Part model, mm, in its own coordinate system. A direction names the side the tool comes from. Coordinates: 2 decimals unless noted, no trailing zeros. Loops run counter-clockwise (first coordinate to the right, second up) from the corner with the lowest first, then second, coordinate; pieces in that order, holes last. Notation, with made-up numbers: (-16, 21.5) - (40, 21.5) arc R23 ccw to (40, 31.5) - close; hole circle Ø11 at (42, 85.5). An arc over 180 degrees is marked (long way). Use a Markdown table: item, result. Add a question column.
1) Tool access for faces 4 (the face through (0, 0, -2)), 5 (the face through (5, 0, -1.27)), 6 (the face through (4, 0, 0)): list every direction of +Z, -Z, +X, -X, +Y, -Y with a clear straight run to the whole face (end or side of a thin tool).
2) Band-saw the part on A-A (z = -2). Give the cut face in (x, y).
3) Drop flat-ended pins along their axis: P1, Ø8, axis at x = 12.5, y = -3, coming from the +Z side; P2, Ø12, axis at x = 4.5, y = 0.5, coming from the -Z side; P3, Ø4, axis at y = -1.5, z = -4, coming from the +X side; P4, Ø4, axis at y = -14.5, z = -3.5, coming from the +X side. Give the stop position or say it passes through.
4) Pull direction Y, two halves, no side cores. Call faces 1 (the face through (-19.05, -1, 4)), 2 (the face through (21.152, -0.864, 0.014)), 3 (the face through (-19.05, 0, -4)): +Y half, -Y half, draft (parallel to the pull), parting line (faces both ways), or undercut.
5) Band-saw the part on B-B (z = 2.5). Give the cut face in (x, y).
6) Probe probe 1 along Y at (x, z) = (16, 1); probe 2 along X at (y, z) = (-1.5, 0.75); probe 3 along Z at (x, y) = (0, 13.5). List the from-to ranges inside material, lowest first. Write a range as [from, to].
from build123d import *

# Parameters (mm, degrees)
F2_R      = 3.6801131425
F3_DEPTH  = 20.32
F4_R      = 4.8020380174
F4_R_2    = 3.6801131425
F5_DEPTH  = 1.27
F6_R      = 4.8020380174
F6_R_2    = 2.3678967055
F7_DEPTH  = 0.762
F9_R      = 21.1697216963
F9_R_2    = 20.3229858377
F10_DEPTH = 1.27
F8_R      = 21.1697216963
F11_DEPTH = 1.27
F12_R     = 0.3048
F13_DEPTH = 0.762


# Not quite as in the source:
# - the program builds the solid bodies; features that only make, move or delete a surface that nothing else refers to are left out


with BuildPart() as f3:
    # F2 (on Right) → F3 (new body)
    with BuildSketch(Plane.YZ):
        Circle(F2_R)
    extrude(amount=-F3_DEPTH)

    # F4 (on face) → F5 (join)
    with BuildSketch(Plane(origin=(-20.32, 0, 0), x_dir=(0, -1, 0), z_dir=(-1, 0, 0))):
        Circle(F4_R)
        Circle(F4_R_2, mode=Mode.SUBTRACT)
    extrude(amount=-F5_DEPTH)

    # F6 (on face) → F7 (join)
    with BuildSketch(Plane(origin=(-20.32, 0, 0), x_dir=(0, -1, 0), z_dir=(-1, 0, 0))):
        Circle(F6_R)
        Circle(F6_R_2, mode=Mode.SUBTRACT)
    extrude(amount=F7_DEPTH)

    # F9 (on face) → F10 (join)
    with BuildSketch(Plane.XY):
        Circle(F9_R)
        Circle(F9_R_2, mode=Mode.SUBTRACT)
    extrude(amount=F10_DEPTH)

    # F8 (on Top) → F11 (join)
    with BuildSketch(Plane.XY):
        Circle(F8_R)
    extrude(amount=-F11_DEPTH)

    # F12
    f12_edges = [f3.edges().sort_by_distance(p)[0] for p in [
        (21.169722, 0, -1.27),
        (21.169722, 0, 1.27),
    ]]
    fillet(f12_edges, radius=F12_R)

    # F13 (add): faces of the model
    f13_faces = [f3.faces().sort_by_distance(p)[0] for p in [
        (-20.32, 0, -1.7192532993),
        (-20.32, 0, 1.4782041027),
    ]]
    extrude(f13_faces, amount=F13_DEPTH)


solid = f3.part
Answer block:
| question | item | result |
|---|---|---|
| 1 | face 4 | -Z, +X, +Y, -Y |
| 1 | face 5 | -Z, +X |
| 1 | face 6 | +Z |
| 2 | outline | (-21.08, -4.37) - (-19.05, -4.37) - (-19.05, -3.09) - (0, -3.09) - (0, 3.09) - (-19.05, 3.09) - (-19.05, 4.37) - (-21.08, 4.37) - close |
| 3 | P1 | z = 0 |
| 3 | P2 | z = -3.68 |
| 3 | P3 | x = 0 |
| 3 | P4 | through |
| 4 | face 1 | undercut |
| 4 | face 2 | parting line |
| 4 | face 3 | draft |
| 5 | outline | (-21.08, -4.1) - (-19.05, -4.1) - (-19.05, -2.7) - (0, -2.7) - (0, 2.7) - (-19.05, 2.7) - (-19.05, 4.1) - (-21.08, 4.1) - close |
| 6 | probe 1 | [-13.86, -12.53], [12.53, 13.86] |
| 6 | probe 2 | [-21.12, 0], [20.27, 21.12] |
| 6 | probe 3 | [-1.27, 0] |
